Autodesk Inventor part; units mm, degrees
ref_plane "YZ Plane" through (0, 0, 0) normal (1, 0, 0) x (0, 1, 0)
ref_plane "XZ Plane" through (0, 0, 0) normal (0, 1, 0) x (-1, 0, 0)
ref_plane "XY Plane" through (0, 0, 0) normal (0, 0, 1) x (1, 0, 0)
sketch "Sketch1" plane through (0, 0, 0) normal (1, 0, 0) x (0, 1, 0)
  arc A0 (1.0277, 65.9115) -> (30.5255, 66.0516) centre (15.7774, 65.8167) ccw
  line L0 (30.5255, 66.0516) -> (30.5255, 81.9568)
  line L1 (40.7755, 78.9568) -> (40.7755, 31.8167)
  circle A1 centre (15.7774, 31.8167) radius 4
  line L2 (-9.2226, 78.8167) -> (-9.2226, 31.8167)
  line L3 (1.0277, 65.9115) -> (1.0277, 81.8167)
  line L4 (-4.2226, 83.8167) -> (-0.9723, 83.8167)
  line L5 (32.5255, 83.9568) -> (35.7755, 83.9568)
  circle A2 centre (0.0401, 32.0007) radius 2.8
  circle A3 centre (31.5401, 32.0007) radius 2.8
  line L6 (15.7774, 31.8167) -> (15.7774, 44.8985) construction
  arc A4 (40.7755, 78.9568) -> (35.7755, 83.9568) centre (35.7755, 78.9568) ccw
  arc A5 (-4.2226, 83.8167) -> (-9.2226, 78.8167) centre (-4.2226, 78.8167) ccw
  line L7 (-4.2226, 26.8167) -> (35.7755, 26.8167)
  arc A6 (-9.2226, 31.8167) -> (-4.2226, 26.8167) centre (-4.2226, 31.8167) ccw
  arc A7 (35.7755, 26.8167) -> (40.7755, 31.8167) centre (35.7755, 31.8167) ccw
  arc A8 (32.5255, 83.9568) -> (30.5255, 81.9568) centre (32.5255, 81.9568) ccw
  arc A9 (1.0277, 81.8167) -> (-0.9723, 83.8167) centre (-0.9723, 81.8167) ccw
  point P0 (-9.2226, 83.8167)
  point P1 (30.5255, 83.9568)
  point P2 (40.7755, 83.9568)
  point P3 (1.0277, 83.8167)
  dimension "d21" = 29.5
  dimension "d44" = 8
  dimension "d57" = 25
  dimension "d64" = 5.6
  dimension "d74" = 18
  dimension "d76" = 5
  dimension "d79" = 2
extrude "Extrusion2" add sketch "Sketch1" along normal blind 6.35
properties part number "motor mount"
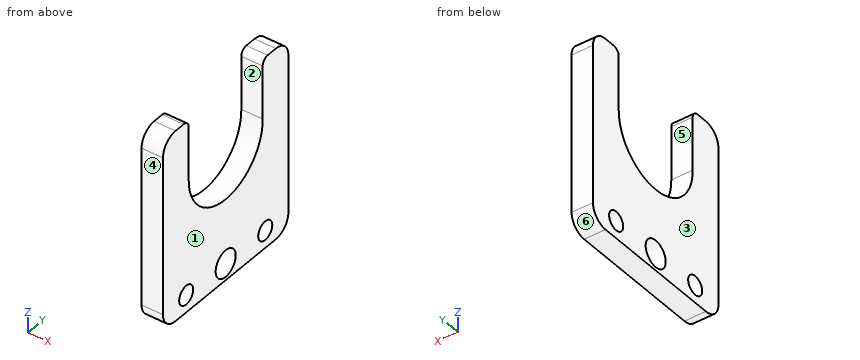
Read the model definition and answer for the solid it produces. Units are mm, in the model's axes. Face numbers are marked on the shaded views. A direction names the side the tool comes from. Give positions to 0.01 mm unless a question says otherwise; leave off trailing zeros. Order: outer loops, then holes, each group sorted by start corner. A loop starts at its lowest first (then second) coordinate and runs counter-clockwise, first axis right, second up. Notation, with made-up numbers: (67.5, 78.5) -> (91.5, 78.5) arc R11 ccw to (91.5, 95.5) -> close; hole circle Ø1 at (18.25, 80.25). An arc over 180 degrees is marked (long way). One line per item, written item: value. Start each with the question number.
(1) Straight lines are drawn through the part: L1, parallel to Y at x = 2.5, z = 74; L2, parallel to Y at x = 2, z = 60; L3, parallel to Y at x = 3, z = 30. For each, find the intervals that lie inside material, in ascending order.
(2) The part is cut by section D-D (y = 24.5). Determine the outline of the cut face in (x, z), and give its area (3 significant figures).
(3) Flat-ended cylindrical pins translate along their axes: P1, Ø3.5, axis at y = 31.54, z = 32, coming from the +X side; P2, Ø1, axis at x = 2.5, y = -2.5, coming from the +Z side. Find the tip coordinate at first contact, or state that the pin passes through.
(4) The part is cut by section C-C (x = 1). Determine the outline of the cut face in (y, z), and give its area (3 significant figures).
(5) The part is cut by section B-B (y = -2). Determine the outline of the cut face in (x, z), and give its area (3 significant figures).
(6) A tool of negligible diameter and unlimited length cuts with its end or side. For the marked faces 1 and 2, from which of +Z, -Z, +X, -X, +Y, -Y can it reach the whole face along a straight path? Write none if from no direction.
(7) The part is cut by section A-A (z = 75.5). Determine the outline of the cut face in (x, y), and give its area (3 significant figures).
(8) For a pull along Y with two mould halves and no side action, classify the marked faces 3, 4, 5 and 6 as released by +Y, released by -Y, zero draft, split by the parting line, or undercut.
Taken from the geometry:
1. L1: -9.22 to 1.03, 30.53 to 40.78
1. L2: -9.22 to 2.22, 29.33 to 40.78
1. L3: -8.88 to -1.92, 2 to 12.21, 19.34 to 29.58, 33.5 to 40.43
2. outline: (0, 26.82) -> (6.35, 26.82) -> (6.35, 53.92) -> (0, 53.92) -> close
2. area: 172 mm^2
3. P1: through
3. P2: z = 83.82
4. outline: (-9.22, 31.82) arc R5 ccw to (-4.22, 26.82) -> (35.78, 26.82) arc R5 ccw to (40.78, 31.82) -> (40.78, 78.96) arc R5 ccw to (35.78, 83.96) -> (32.53, 83.96) arc R2 ccw to (30.53, 81.96) -> (30.53, 66.05) arc R14.75 cw (long way) to (1.03, 65.91) -> (1.03, 81.82) arc R2 ccw to (-0.97, 83.82) -> (-4.22, 83.82) arc R5 ccw to (-9.22, 78.82) -> close; hole circle Ø5.6 at (0.04, 32); hole circle Ø8 at (15.78, 31.82); hole circle Ø5.6 at (31.54, 32)
4. area: 1,860 mm^2
5. outline: (0, 26.82) -> (6.35, 26.82) -> (6.35, 30.08) -> (0, 30.08) -> close; (0, 33.92) -> (6.35, 33.92) -> (6.35, 83.82) -> (0, 83.82) -> close
5. area: 338 mm^2
6. face 1: +Z, -Z, +X, +Y, -Y
6. face 2: +Z, +X, -X
7. outline: (0, -9.22) -> (6.35, -9.22) -> (6.35, 1.03) -> (0, 1.03) -> close; (0, 30.53) -> (6.35, 30.53) -> (6.35, 40.78) -> (0, 40.78) -> close
7. area: 130 mm^2
8. face 3: zero draft
8. face 4: released by -Y
8. face 5: undercut
8. face 6: released by +Y
